Autodesk Inventor part; units mm, degrees
ref_plane "YZ Plane" through (0, 0, 0) normal (1, 0, 0) x (0, 1, 0)
ref_plane "XZ Plane" through (0, 0, 0) normal (0, 1, 0) x (-1, 0, 0)
ref_plane "XY Plane" through (0, 0, 0) normal (0, 0, 1) x (1, 0, 0)
sketch "Sketch1" plane through (0, 0, 0) normal (0, 0, 1) x (1, 0, 0)
  line L0 (0, 0) -> (19.05, 0)
  line L1 (19.05, 0) -> (19.05, 44.45)
  line L2 (19.05, 44.45) -> (0, 44.45)
  line L3 (0, 44.45) -> (0, 0)
  line L4 (19.05, 44.45) -> (6.35, 44.45)
  line L5 (6.35, 44.45) -> (6.35, 15.875)
  line L6 (9.525, 12.7) -> (19.05, 12.7)
  line L7 (19.05, 12.7) -> (19.05, 44.45)
  arc A0 (6.35, 15.875) -> (9.525, 12.7) centre (9.525, 15.875) ccw
  point P0 (6.35, 12.7)
  dimension "d0" = 44.45
  dimension "d1" = 19.05
  dimension "d2" = 31.75
  dimension "d3" = 6.35
  dimension "d4" = 3.175
extrude "Extrusion1" add sketch "Sketch1" along normal blind 25.4 contours L3 L2 L5 A0 L6 L1 L0
sketch "Sketch2" plane through (0, 0, 0) normal (-1, 0, 0) x (0, 0, 1)
  line L0 (0, 44.45) -> (25.4, 44.45)
  point P0 (12.7, 38.1)
  point P1 (12.7, 25.4)
  point P2 (12.7, 44.45)
  dimension "d7" = 12.7
  dimension "d8" = 6.35
hole "Hole1" at (0, 38.1, 12.7) at (0, 25.4, 12.7) direction (1, 0, 0) diameter 5.1054 end through all
sketch "Sketch3" plane through (0, 0, 0) normal (-1, 0, 0) x (0, 0, 1)
  line L0 (0, 0) -> (25.4, 0)
  line L1 (6.35, 0) -> (19.05, 0)
  line L2 (19.05, 0) -> (19.05, 7.62)
  line L3 (19.05, 7.62) -> (6.35, 7.62)
  line L4 (6.35, 7.62) -> (6.35, 0)
  point P0 (12.7, 0)
  dimension "d16" = 12.7
  dimension "d17" = 7.62
extrude "Extrusion2" cut sketch "Sketch3" against normal through all
properties part number "gripper jaw"
Here's how the part is built. I have some questions about the finished solid (model axes, mm). A direction names the side the tool comes from. Round coordinates to 2 decimals unless told otherwise and drop trailing zeros. Write each loop counter-clockwise with the first axis right and the second up, starting at its lowest first coordinate (ties: lowest second). Pieces come first, ordered by that corner, then holes. Notation, with made-up numbers: M -37.75,27 L 4.25,27 A17 cw 4.25,52 Z; hole C 72,-17 d3. An arc over 180 degrees is marked long. Answer as CSV lines item,"result". Start each with the question number.
1. I need wall thicknesses on probe 1 along Y at (x, z) = (2.5, 12.7); probe 2 along Z at (x, y) = (1.5, 38.1); probe 3 along Y at (x, z) = (16, 15.75). Which ranges of each line are inside material? Lowest first, please.
2. Suppose I cut it at A-A on y = 6. Write out the boundary of the cut face in (x, z), then the cut area to 3 significant figures.
3. On a 3-axis mill with a long thin cutter (end or side, diameter ignored), from which of +Z, -Z, +X, -X, +Y, -Y can I reach the whole of each face in a straight line? I mean faces 1 (the flat face through (9, 4, 6.35)), 2 (the flat face through (14, 12.7, 13)), 3 (the flat face through (9, 0, 3)). Say none if no direction works.
4. Suppose I cut it at D-D on z = 21.5. Write out the boundary of the cut face in (x, y) (3 decimals).
5. Suppose I cut it at B-B on z = 12.7. Write out the boundary of the cut face in (x, y) (3 decimals), then the cut area to 3 significant figures.
6. Suppose I cut it at C-C on x = 5.25. Write out the boundary of the cut face in (y, z).
7. Thinking about a two-plate mould opening in Z: for faces 4 (the flat face through (9, 0, 22)), 5 (the flat face through (5, 18, 0)), 6 (the cylindrical face through (3.219, 26.378, 15.058)), which applies, released by +Z, released by -Z, zero draft, split by the parting line, or undercut?
8. I'm going to push flat-ended pins straight in: pin 1 Ø5 at (x, z) = (15, 6.5) entering from +Y; pin 2 Ø5 at (y, z) = (27, 22) entering from +X; pin 3 Ø8 at (y, z) = (33.5, 21) entering from -X; pin 4 Ø4.5 at (y, z) = (25.4, 12.7) entering from -X. Where does each tip first touch, or does it pass through?
Check result:
1,probe 1,"y = 7.62 to 22.85, 27.95 to 35.55, 40.65 to 44.45"
1,probe 2,"z = 0 to 10.15, 15.25 to 25.4"
1,probe 3,"y = 7.62 to 12.7"
2,outline,"M 0,0 L 19.05,0 L 19.05,6.35 L 0,6.35 Z; M 0,19.05 L 19.05,19.05 L 19.05,25.4 L 0,25.4 Z"
2,area,"242 mm2"
3,face 1,"+X, -X, -Y"
3,face 2,"+Z, -Z, +X, +Y"
3,face 3,"+Z, -Z, +X, -X, -Y"
4,outline,"M 0,0 L 19.05,0 L 19.05,12.7 L 9.525,12.7 A3.175 cw 6.35,15.875 L 6.35,44.45 L 0,44.45 Z"
5,outline,"M 0,7.62 L 19.05,7.62 L 19.05,12.7 L 9.525,12.7 A3.175 cw 6.35,15.875 L 6.35,22.847 L 0,22.847 Z; M 0,27.953 L 6.35,27.953 L 6.35,35.547 L 0,35.547 Z; M 0,40.653 L 6.35,40.653 L 6.35,44.45 L 0,44.45 Z"
5,area,"236 mm2"
6,outline,"M 0,0 L 44.45,0 L 44.45,25.4 L 0,25.4 L 0,19.05 L 7.62,19.05 L 7.62,6.35 L 0,6.35 Z; hole C 25.4,12.7 d5.11; hole C 38.1,12.7 d5.11"
7,face 4,"zero draft"
7,face 5,"released by -Z"
7,face 6,"undercut"
8,pin 1,"stops at y = 12.7"
8,pin 2,"stops at x = 6.35"
8,pin 3,"stops at x = 0"
8,pin 4,"passes through"
